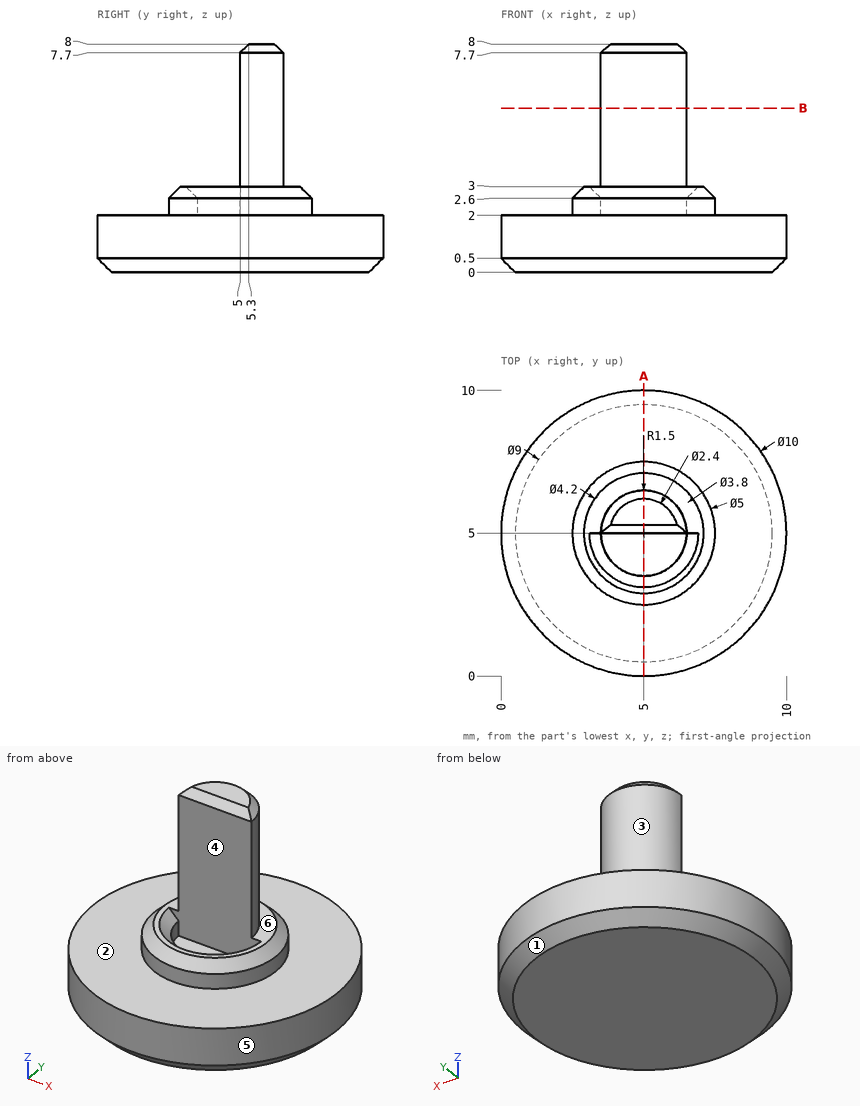
The drawing under review shows one solid part. Ordinate dimensions are in mm from its lowest x, y, z. A direction names the side the tool comes from. Round coordinates to 2 decimals unless told otherwise and drop trailing zeros. Write each loop counter-clockwise with the first axis right and the second up, starting at its lowest first coordinate (ties: lowest second). Pieces come first, ordered by that corner, then holes. Notation, with made-up numbers: (-0.75, -7.75) - (4.25, -7.75) arc R13 cw to (4.25, -3.75) - close; hole circle Ø2 at (80, -26). An arc over 180 degrees is marked (long way). Use one line per item in the form item = value.
Q1. Draft analysis for pull direction Y (two halves, no side actions). For the marked faces 3, 4, 5 and 6, state which applies: +Y half, -Y half, draft (parallel to the pull), parting line (faces both ways), or undercut.
Answer key:
face_3 = +Y half
face_4 = undercut
face_5 = parting line
face_6 = draft
Q2. Tool access review of the marked faces 1 and 2: name each direction out of +Z, -Z, +X, -X, +Y, -Y from which nothing blocks a thin tool from reaching the whole face with its end or side.
Answer key:
face_1 = -Z
face_2 = +Z
Q3. Consider section A-A (x = 5). State the section outline as (y, z) points.
Answer key:
outline = (0, 0.5) - (0.5, 0) - (9.5, 0) - (10, 0.5) - (10, 2) - (7.5, 2) - (7.5, 2.6) - (7.1, 3) - (6.5, 3) - (6.5, 7.7) - (6.2, 8) - (5.3, 8) - (5, 7.7) - (5, 2) - (3.5, 2) - (3.5, 2.6) - (3.1, 3) - (2.9, 3) - (2.5, 2.6) - (2.5, 2) - (0, 2) - close
Q4. For line 1 (Z direction, x = 1.75, y = 7.5); line 2 (Z direction, x = 7, y = 5); line 3 (X direction, y = 4.25, z = 2.25), list the stretches that pass through material, from the lowest coordinate up. Write a range as [from, to].
Answer key:
line_1 = [0, 2]
line_2 = [0, 3]
line_3 = [2.62, 3.7], [6.3, 7.38]
Q5. Insertion check: pin 1 Ø2 at (x, y) = (8, 3.5) entering from +Z; pin 2 Ø1.9 at (x, z) = (5.5, 6) entering from -Y; pin 3 Ø2 at (x, y) = (8.5, 4.5) entering from +Z; pin 4 Ø1.5 at (x, z) = (2, 4) entering from -Y. Each pin has a flat end and moves straight along its axis. Give the tip position at first contact, or say it passes through.
Answer key:
pin_1 = 2.75
pin_2 = 5
pin_3 = 2
pin_4 = through
Q6. Consider section B-B (z = 5.75). State the section outline as (x, y) points.
Answer key:
outline = (3.5, 5) - (6.5, 5) arc R1.5 ccw to start
